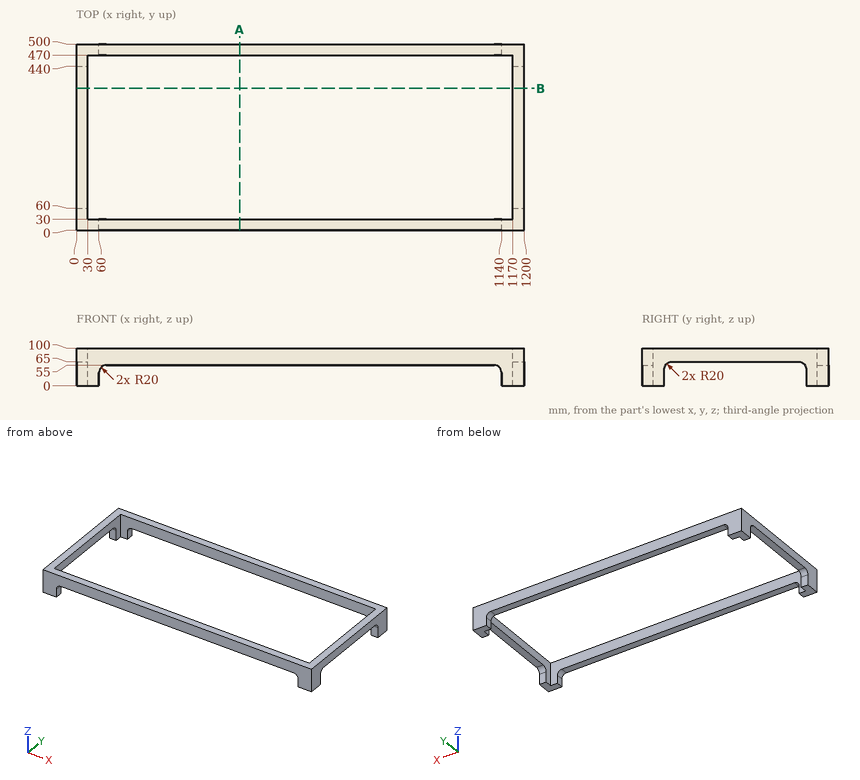
Drawing for the job (mm, zero at the part's lowest x, y, z). Round coordinates to 2 decimals unless told otherwise and drop trailing zeros. Write each loop counter-clockwise with the first axis right and the second up, starting at its lowest first coordinate (ties: lowest second). Pieces come first, ordered by that corner, then holes. Notation, with made-up numbers: (-31.75, 52.25) - (-7.75, 52.25) arc R10 ccw to (-7.75, 65.25) - close; hole circle Ø1 at (84.25, 17.25). An arc over 180 degrees is marked (long way). Return JSON: item names as keys, results as strings. Group by question number.
Item 1: Flat gauge pin, fed straight in: pin 1 Ø24 at (x, y) = (742.5, 17) entering from -Z. Where does the tip first touch, or does it go through?
Item 2: Band-saw the part on A-A on x = 437.5. List the corners of the cut face in (y, z).
Item 3: Probe probe 1 along Y at (x, z) = (650.5, 96); probe 2 along X at (y, z) = (68, 78.5). List the from-to ranges inside material, lowest first.
Item 4: Band-saw the part on B-B on y = 381. List the corners of the cut face in (x, z), plus the area to 3 significant figures.
Resolved:
{
 "1": {"pin 1": "stops at z = 55"},
 "2": {"outline": "(0, 55) - (30, 55) - (30, 100) - (0, 100) - close; (470, 55) - (500, 55) - (500, 100) - (470, 100) - close"},
 "3": {"probe 1": "y = 0 to 30, 470 to 500", "probe 2": "x = 0 to 30, 1170 to 1200"},
 "4": {"outline": "(0, 65) - (30, 65) - (30, 100) - (0, 100) - close; (1170, 65) - (1200, 65) - (1200, 100) - (1170, 100) - close", "area": "2,100 mm²"}
}
